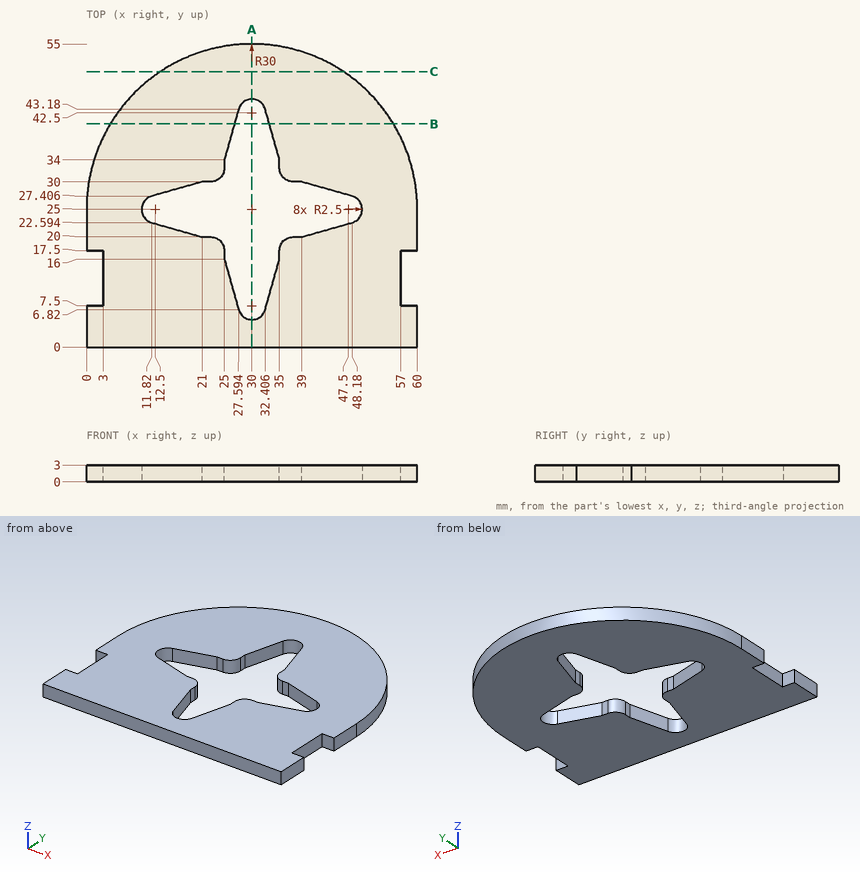
Print and shaded views of the part. All mm, measured from the part's lowest x, y and z. Coordinates: 2 decimals unless noted, no trailing zeros. Order: outer loops, then holes, each group sorted by start corner. A loop starts at its lowest first (then second) coordinate and runs counter-clockwise, first axis right, second up. Notation, with made-up numbers: M -13.75,-35 L 16.25,-35 A23 cw 16.25,-19 Z; hole C -9.5,-19.5 d3. An arc over 180 degrees is marked long. Write each question's results on one line, items separated by ' | '. Start each with the question number.
Q1. Cut at C-C (y = 50). List the corners of the cut face in (x, z).
Q2. Cut at B-B (y = 40.5). List the corners of the cut face in (x, z), then the cut area to 3 significant figures.
Q3. Drill centre lines: probe 1 along Y at (x, z) = (30, 2.6); probe 2 along X at (y, z) = (16, 1.15); probe 3 along Y at (x, z) = (15, 0.75) (1 decimal). Where is each one in solid material? Low to high. Write a range as from..to.
Q4. Cut at A-A (x = 30). List the corners of the cut face in (y, z), then the cut area to 3 significant figures.
Q5. Flat gauge pins, fed straight in: P1, Ø1.2, axis at x = 22, z = 1.5, coming from the -Y side; P2, Ø1.6, axis at y = 33.5, z = 2, coming from the -X side (3 decimals); P3, Ø1.2, axis at y = 33.5, z = 1, coming from the +X side; P4, Ø1, axis at y = 33.5, z = 1.5, coming from the -X side. Where does each tip first touch, or does it go through?
Found:
1) outline: M 13.42,0 L 46.58,0 L 46.58,3 L 13.42,3 Z
2) outline: M 4.31,0 L 26.84,0 L 26.84,3 L 4.31,3 Z; M 33.16,0 L 55.69,0 L 55.69,3 L 33.16,3 Z | area: 135 mm²
3) probe 1: 0..5, 45..55 | probe 2: 3..25, 35..57 | probe 3: 0..21.7, 28.3..51
4) outline: M 0,0 L 5,0 L 5,3 L 0,3 Z; M 45,0 L 55,0 L 55,3 L 45,3 Z | area: 45.0 mm²
5) P1: y = 0 | P2: x = 1.005 | P3: x = 58.94 | P4: x = 1.09
